Geometry check sheet. Reference: the model listing, model coordinates, mm. A direction names the side the tool comes from. Round coordinates to 2 decimals unless told otherwise and drop trailing zeros. Write each loop counter-clockwise with the first axis right and the second up, starting at its lowest first coordinate (ties: lowest second). Pieces come first, ordered by that corner, then holes. Notation, with made-up numbers: (85.5, 19) - (129.5, 19) arc R23 ccw to (129.5, 40) - close; hole circle Ø2 at (-20, 35.25). An arc over 180 degrees is marked (long way). Return JSON: item names as keys, results as strings.
Autodesk Inventor part; units mm, degrees
ref_plane "YZ Plane" through (0, 0, 0) normal (1, 0, 0) x (0, 1, 0)
ref_plane "XZ Plane" through (0, 0, 0) normal (0, 1, 0) x (-1, 0, 0)
ref_plane "XY Plane" through (0, 0, 0) normal (0, 0, 1) x (1, 0, 0)
sketch "Sketch1" plane through (0, 0, 0) normal (1, 0, 0) x (0, 1, 0)
  line L0 (266.7, 158.75) -> (-266.7, 158.75)
  line L1 (-266.7, 158.75) -> (-266.7, -158.75)
  line L2 (-266.7, -158.75) -> (266.7, -158.75)
  line L3 (266.7, -158.75) -> (266.7, 158.75)
  line L4 (266.7, 158.75) -> (-266.7, -158.75) construction
  line L5 (-266.7, 158.75) -> (266.7, -158.75) construction
  point P0 (0, 0)
  dimension "d0" = 533.4
  dimension "d1" = 317.5
extrude "Extrusion1" add sketch "Sketch1" along normal blind 20.32
sketch "Sketch2" plane through (20.32, 0, 0) normal (1, 0, 0) x (0, 0, -1)
  line L0 (-158.75, 266.7) -> (-158.75, -266.7)
  line L1 (158.75, 266.7) -> (-158.75, 266.7)
  line L2 (-158.75, -266.7) -> (-140.97, -266.7)
  line L3 (-140.97, -266.7) -> (-140.97, 266.7)
  line L4 (-140.97, 266.7) -> (-158.75, 266.7)
  line L5 (-158.75, 266.7) -> (-158.75, -266.7)
  line L6 (158.75, 266.7) -> (-140.97, 266.7)
  line L7 (-140.97, 266.7) -> (-140.97, -266.7)
  line L8 (-140.97, -266.7) -> (158.75, -266.7)
  line L9 (158.75, -266.7) -> (158.75, 266.7)
  point P0 (0, 0)
  dimension "d4" = 17.78
extrude "Extrusion2" cut sketch "Sketch2" against normal blind 2.54 contours L1 L9 L8 L3
sketch "Sketch3" plane through (17.78, 0, 0) normal (1, 0, 0) x (0, 0, -1)
  line L0 (-140.97, -266.7) -> (-140.97, 266.7)
  line L1 (-140.97, 266.7) -> (-140.97, 256.54)
  line L2 (-140.97, -266.7) -> (-140.97, -256.54)
  line L3 (158.75, -266.7) -> (158.75, 266.7)
  line L4 (158.75, 0) -> (148.59, 0)
  line L5 (-140.97, -256.54) -> (148.59, -256.54)
  line L6 (148.59, -256.54) -> (148.59, 256.54)
  line L7 (148.59, 256.54) -> (-140.97, 256.54)
  line L8 (-140.97, 256.54) -> (-140.97, -256.54)
  point P0 (0, 0)
  dimension "d7" = 10.16
  dimension "d8" = 10.16
  dimension "d9" = 10.16
extrude "Extrusion3" cut sketch "Sketch3" against normal blind 5.08
sketch "Sketch4" plane through (0, -266.7, 158.75) normal (0, 0, 1) x (1, 0, 0)
  line L0 (0, 266.7) -> (-30.48, 266.7)
  line L1 (-30.48, 266.7) -> (-30.48, 393.7)
  line L2 (-30.48, 266.7) -> (-30.48, 139.7)
  line L3 (0, 0) -> (20.32, 0)
  spline S0 degree 2 poles (0, 0) (-29.2196, 51.877) (-30.48, 139.7) knots 0 0 0 1 1 1
  spline S1 degree 2 poles (0, 533.4) (-29.2196, 481.523) (-30.48, 393.7) knots 0 0 0 1 1 1
  line L4 (0, 0) -> (0, 533.4)
  line L5 (20.32, 533.4) -> (20.32, 0)
  point P0 (-20.6375, 53.975)
  point P1 (-20.6375, 479.425)
  dimension "d12" = 30.48
  dimension "d13" = 127
  dimension "d14" = 127
extrude "Extrusion4" add sketch "Sketch4" against normal blind 317.5
sketch "Sketch5" plane through (17.78, 266.7, 140.97) normal (0, 1, 0) x (1, 0, 0)
  line L0 (-17.78, 299.72) -> (0, 299.72)
  line L1 (-48.26, -17.78) -> (-48.26, 299.72)
  spline S0 degree 2 poles (-17.78, 299.72) (-47.3289, 249.7338) (-48.26, 184.15) knots 0 0 0 1 1 1
  line L2 (-48.26, 184.15) -> (-48.26, 299.72)
  line L3 (-48.26, 299.72) -> (-17.78, 299.72)
  point P0 (-17.78, 140.97)
  point P1 (-39.6875, 247.65)
extrude "Extrusion5" cut sketch "Sketch5" against normal blind 533.4
fillet "Fillet1" radius 3.81 4 edges at (8.89, 266.7, -158.75) (8.89, -266.7, -158.75) (10.16, -266.7, 158.75) (10.16, 266.7, 158.75)
fillet "Fillet2" radius 1.27 2 edges at (15.24, -256.54, -148.59) (15.24, 256.54, -148.59)
chamfer "Chamfer1" distance 1.27 angle 45 5 edges at (17.78, 256.54, -3.175) (17.78, 256.168, -148.218) (17.78, 0, -148.59) (17.78, -256.168, -148.218) (17.78, -256.54, -3.175)
sketch "Sketch6" plane through (-30.48, -127, 158.75) normal (0, 0, 1) x (1, 0, 0)
  line L0 (0, 0) -> (0, 254)
  line L1 (0, 127) -> (30.48, 127)
  line L2 (30.48, 127) -> (30.48, 228.6)
  line L3 (30.48, 127) -> (30.48, 25.4)
  line L4 (0, 127) -> (0, 304.8)
  line L5 (0, 127) -> (0, -50.8)
  spline S0 degree 2 poles (0, -50.8) (21.577, -20.7599) (30.48, 25.4) knots 0 0 0 1 1 1
  spline S1 degree 2 poles (0, 304.8) (21.577, 274.7599) (30.48, 228.6) knots 0 0 0 1 1 1
  point P0 (17.4625, -19.05)
  point P1 (17.4625, 273.05)
  dimension "d24" = 101.6
  dimension "d25" = 101.6
  dimension "d26" = 177.8
  dimension "d27" = 177.8
extrude "Extrusion6" cut sketch "Sketch6" against normal blind 78.74
fillet "Fillet3" radius 127 2 edges at (0, -101.6, 119.38) (0, 101.6, 119.38)
sketch "Sketch7" plane through (0, 266.7, 154.94) normal (0, 1, 0) x (1, 0, 0)
  line L0 (-2.0826, -3.81) -> (20.32, -3.81)
  line L1 (0, -3.81) -> (0, 12.7)
  line L2 (0, 12.7) -> (-10.16, 12.7)
  line L3 (-10.16, 12.7) -> (-10.16, 58.42)
  line L4 (-10.16, 58.42) -> (0, 58.42)
  line L5 (0, 58.42) -> (0, 12.7)
  point P0 (0, 154.94)
  dimension "d31" = 16.51
  dimension "d32" = 10.16
  dimension "d33" = 45.72
extrude "Extrusion7" add sketch "Sketch7" against normal blind 65.7225
fillet "Fillet4" radius 25.4 1 edges at (-10.16, 245.5271, 120.309)
sketch "Sketch8" plane through (-30.48, -127, -43.18) normal (-1, 0, 0) x (0, 0, 1)
  line L0 (123.19, 214.5104) -> (123.19, 39.4896)
  line L1 (123.19, 127) -> (85.09, 127)
  line L2 (85.09, 127) -> (38.1, 127)
  circle A0 centre (38.1, 127) radius 46.99
  point P0 (43.18, 127)
  dimension "d37" = 38.1
  dimension "d38" = 46.99
  dimension "d39" = 93.98
extrude "Extrusion8" add sketch "Sketch8" against normal blind 7.9375
extrude "Extrusion9" add sketch "Sketch8" along normal blind 44.45
properties part number "DellP2317H" material "ABS Plastic"
(1) Gauge pin test, flat ends, axial feed: pin 1 (2 mm diameter, centred on y = 106, z = 66, fed in from -X); pin 2 (2 mm diameter, centred on x = -5.5, y = 29, fed in from -Z); pin 3 (5 mm diameter, centred on x = -18, y = 32.5, fed in from +Z). Record the tip position at first contact, or that the pin passes through.
Response values:
{"pin 1": "stops at x = -30.48", "pin 2": "stops at z = -150.74", "pin 3": "stops at z = 80.01"}
(2) Access from +Z, -Z, +X, -X, +Y, -Y to the whole of each face (thin tool, end or side, straight path). Record for faces 1 (the face through (0, 1, 120)), 2 (the face through (12.7, 4, -2)), 3 (the face through (17.78, 120, -153)), 4 (the face through (10, -266.7, 2)), 5 (the face through (-10.16, 259, 120)).
Response values:
{"face 1": "+Z, -X", "face 2": "+X", "face 3": "-Z, +X, +Y, -Y", "face 4": "+Z, -Z, +X, -X, -Y", "face 5": "+Z, -Z, -X, +Y"}
(3) Section check A-A, the plane x = -37. Enter the section's corners in (y, z), plus the area to 3 significant figures.
Response values:
{"outline": "circle Ø93.98 at (0, -5.08)", "area": "6,940 mm^2"}
(4) Material ranges on line 1 along Z through (x, y) = (14, -76.5); line 2 along X through (y, z) = (-127.5, -28); line 3 along X through (y, z) = (15.5, -9.5), recorded low to high. Write a range as [from, to].
Response values:
{"line 1": "z = [-158.75, -148.59], [140.97, 158.75]", "line 2": "x = [-30.47, 12.7]", "line 3": "x = [-74.93, 12.7]"}
(5) Release check for a two-part mould opening along Y. For faces 6 (the face through (8, 266.7, -2)), 7 (the face through (-52.26, 28.59, -42.37)), 8 (the face through (1, 4, 158.75)), 9 (the face through (-15, 2, 80.01)) record: pulls with the +Y half, pulls with the -Y half, needs draft (parallel to the pull), parting line crosses it, or undercut.
Response values:
{"face 6": "pulls with the +Y half", "face 7": "parting line crosses it", "face 8": "needs draft", "face 9": "undercut"}
